Source: CAD feature listing. Evaluate the final solid. Frame: model axes, mm. Face numbers are marked on the shaded views. Round coordinates to 2 decimals unless told otherwise and drop trailing zeros. Loops run counter-clockwise (first coordinate to the right, second up) from the corner with the lowest first, then second, coordinate; pieces in that order, holes last. Notation, with made-up numbers: (4, 20.5) -> (52, 20.5) arc R15 ccw to (52, 26.5) -> close; hole circle Ø11 at (-38.75, -14.75). An arc over 180 degrees is marked (long way). Write item = value, one per line.
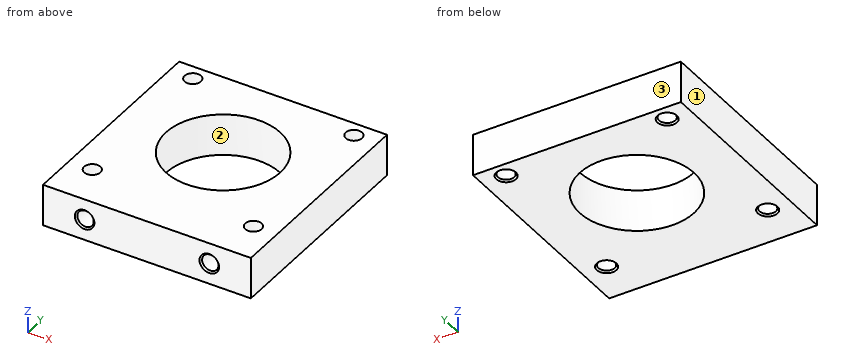
from build123d import *

# Parameters (mm, degrees)
ESBO_O1_W                                         = 40
ESBO_O1_H                                         = 42
RESSALTO_EXTRUS_O1_DEPTH                          = 8
ESBO_O2_R                                         = 11
CORTE_EXTRUS_O1_DEPTH                             = 9
FURO_ROSCADO_PARA_CONDU_TE_DE_M3X0_51_D           = 3.15
FURO_ROSCADO_PARA_CONDU_TE_DE_M3X0_51_DEPTH       = 10
FURO_ROSCADO_PARA_CONDU_TE_DE_M3X0_51_CSINK_D     = 3.766
FURO_ROSCADO_PARA_CONDU_TE_DE_M3X0_51_CSINK_ANGLE = 90
FURO_ROSCADO_PARA_CONDU_TE_DE_M3X0_51_TIP         = 0.946355475
FURO_ROSCADO_PARA_CONDU_TE_DE_M3X0_52_D           = 3.15
FURO_ROSCADO_PARA_CONDU_TE_DE_M3X0_52_CSINK_D     = 3.766
FURO_ROSCADO_PARA_CONDU_TE_DE_M3X0_52_CSINK_ANGLE = 90


with BuildPart() as part:
    # Esboço1 → Ressalto-extrusão1 (new body)
    with BuildSketch(Plane.XY):
        Rectangle(ESBO_O1_W, ESBO_O1_H)
    extrude(amount=RESSALTO_EXTRUS_O1_DEPTH)

    # Esboço2 → Corte-extrusão1 (cut, through all)
    with BuildSketch(Plane.XY.offset(8)):
        with Locations((0, 2.5)):
            Circle(ESBO_O2_R)
    extrude(amount=-CORTE_EXTRUS_O1_DEPTH, mode=Mode.SUBTRACT)

    # Furo roscado para conduíte de M3x0.51
    with Locations(Plane(origin=(0, -21, 0), x_dir=(-1, 0, 0), z_dir=(0, -1, 0))):
        with Locations((-12, -4), (12, -4)):
            CounterSinkHole(FURO_ROSCADO_PARA_CONDU_TE_DE_M3X0_51_D / 2, FURO_ROSCADO_PARA_CONDU_TE_DE_M3X0_51_CSINK_D / 2, depth=FURO_ROSCADO_PARA_CONDU_TE_DE_M3X0_51_DEPTH, counter_sink_angle=FURO_ROSCADO_PARA_CONDU_TE_DE_M3X0_51_CSINK_ANGLE)
            with Locations((0, 0, -(FURO_ROSCADO_PARA_CONDU_TE_DE_M3X0_51_DEPTH + FURO_ROSCADO_PARA_CONDU_TE_DE_M3X0_51_TIP / 2))):  # 118° drill point
                Cone(0, FURO_ROSCADO_PARA_CONDU_TE_DE_M3X0_51_D / 2, FURO_ROSCADO_PARA_CONDU_TE_DE_M3X0_51_TIP, mode=Mode.SUBTRACT)

    # Furo roscado para conduíte de M3x0.52 (through all)
    with Locations(Plane(origin=(0, 0, 0), x_dir=(-1, 0, 0), z_dir=(0, 0, -1))):
        with Locations((-15.5, 18), (15.5, 18), (-15.5, -13), (15.5, -13)):
            CounterSinkHole(FURO_ROSCADO_PARA_CONDU_TE_DE_M3X0_52_D / 2, FURO_ROSCADO_PARA_CONDU_TE_DE_M3X0_52_CSINK_D / 2, counter_sink_angle=FURO_ROSCADO_PARA_CONDU_TE_DE_M3X0_52_CSINK_ANGLE)


solid = part.part
1. Mould query, pull axis Y, two halves, no side actions, for the marked faces 1, 2 and 3. Classes: released by +Y, released by -Y, zero draft, split by the parting line, or undercut.
Evaluation:
face_1 = zero draft
face_2 = undercut
face_3 = released by +Y
2. Section query C-C (y = 2.5). Return the cut outline in (x, z).
Evaluation:
outline = (-20, 0) -> (-11, 0) -> (-11, 8) -> (-20, 8) -> close; (11, 0) -> (20, 0) -> (20, 8) -> (11, 8) -> close
3. Line query: probe 1 along Y at (x, z) = (-15.5, 2.75) (3 decimals); probe 2 along X at (y, z) = (-17.75, 4) (3 decimals); probe 3 along X at (y, z) = (-13, 2) (3 decimals). Output: solid intervals per line, ascending. Write a range as from..to.
Evaluation:
probe_1 = -21..-14.575, -11.425..16.425, 19.575..21
probe_2 = -20..-13.575, -10.425..10.425, 13.575..20
probe_3 = -20..-17.075, -13.925..13.925, 17.075..20
4. Section query A-A (y = -13). Return the cut outline in (x, z) (3 decimals), then the cut area to 3 significant figures.
Evaluation:
outline = (-20, 0) -> (-17.383, 0) -> (-17.075, 0.308) -> (-17.075, 8) -> (-20, 8) -> close; (-13.925, 0.308) -> (-13.617, 0) -> (13.617, 0) -> (13.925, 0.308) -> (13.925, 8) -> (-13.925, 8) -> close; (17.075, 0.308) -> (17.383, 0) -> (20, 0) -> (20, 8) -> (17.075, 8) -> close; hole circle Ø3.15 at (-12, 4); hole circle Ø3.15 at (12, 4)
area = 254 mm²
5. Section query D-D (y = 18). Return the cut outline in (x, z) (3 decimals).
Evaluation:
outline = (-20, 0) -> (-17.383, 0) -> (-17.075, 0.308) -> (-17.075, 8) -> (-20, 8) -> close; (-13.925, 0.308) -> (-13.617, 0) -> (13.617, 0) -> (13.925, 0.308) -> (13.925, 8) -> (-13.925, 8) -> close; (17.075, 0.308) -> (17.383, 0) -> (20, 0) -> (20, 8) -> (17.075, 8) -> close
6. Section query B-B (z = 7.25). Return the cut outline in (x, y) (3 decimals).
Evaluation:
outline = (-20, -21) -> (20, -21) -> (20, 21) -> (-20, 21) -> close; hole circle Ø3.15 at (-15.5, -13); hole circle Ø3.15 at (-15.5, 18); hole circle Ø22 at (0, 2.5); hole circle Ø3.15 at (15.5, -13); hole circle Ø3.15 at (15.5, 18)
